Verification items for this drawing (mm, ordinates from the low corner). A direction names the side the tool comes from. Coordinates: 2 decimals unless noted, no trailing zeros. Write each loop counter-clockwise with the first axis right and the second up, starting at its lowest first coordinate (ties: lowest second). Pieces come first, ordered by that corner, then holes. Notation, with made-up numbers: (-6, 78.25) -> (17, 78.25) arc R24 ccw to (17, 117.25) -> close; hole circle Ø6 at (44.5, -10.5). An arc over 180 degrees is marked (long way). One line per item, written item: value. Start each with the question number.
1) Scan lines: line 1 along Z through (x, y) = (4.25, 5.5); line 2 along Z through (x, y) = (5.25, 1); line 3 along Z through (x, y) = (5, 7). Record each from-to range of solid material in increasing order. Write a range as [from, to].
2) Set-up check for the marked faces 1, 2 and 3: record each of +Z, -Z, +X, -X, +Y, -Y from which the full face is reachable in a straight line by a thin tool's end or side.
3) Sectioned sample at D-D on z = 13. Enter the section's corners in (x, y), plus the area to 3 significant figures.
4) Sectioned sample at A-A on x = 4. Enter the section's corners in (y, z), plus the area to 3 significant figures.
5) Sectioned sample at C-C on z = 18.25. Enter the section's corners in (x, y).
6) Gauge pin test, flat ends, axial feed: P1, Ø2, axis at x = 1, y = 4.5, coming from the -Z side; P2, Ø4, axis at x = 2.5, z = 6.5, coming from the +Y side. Record the tip position at first contact, or that the pin passes through.
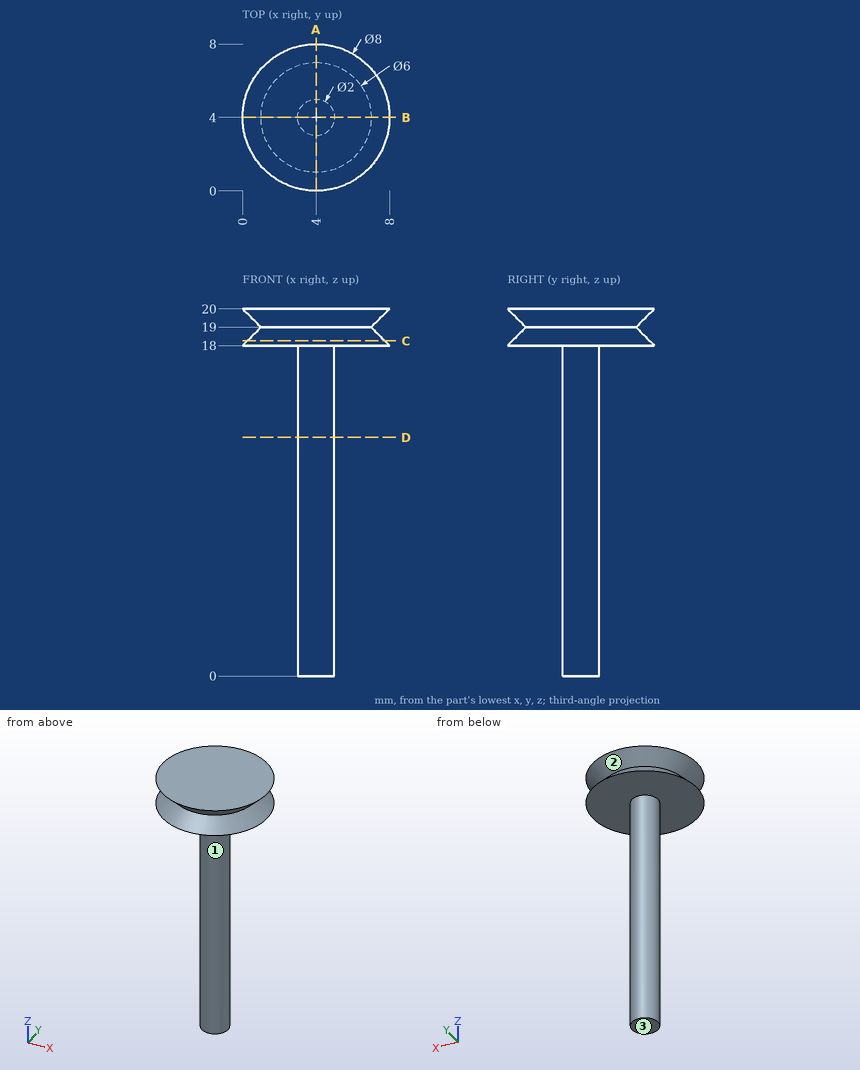
Answers:
1. line 1: z = [18, 20]
1. line 2: z = [18, 18.75], [19.25, 20]
1. line 3: z = [18, 18.84], [19.16, 20]
2. face 1: -Z
2. face 2: none
2. face 3: -Z, +X, -X, +Y, -Y
3. outline: circle Ø2 at (4, 4)
3. area: 3.14 mm2
4. outline: (0, 18) -> (3, 18) -> (3, 0) -> (5, 0) -> (5, 18) -> (8, 18) -> (7, 19) -> (8, 20) -> (0, 20) -> (1, 19) -> close
4. area: 50.0 mm2
5. outline: circle Ø7.5 at (4, 4)
6. P1: stops at z = 18
6. P2: stops at y = 5
